For this review, take the finished solid that the model builds, in its own axes (mm). Face numbers are marked on the shaded views. A direction names the side the tool comes from. Give positions to 0.01 mm unless a question says otherwise; leave off trailing zeros. Write each loop counter-clockwise with the first axis right and the second up, starting at its lowest first coordinate (ties: lowest second). Pieces come first, ordered by that corner, then holes. Notation, with made-up numbers: M -31.75,33.5 L -14.75,33.5 A30 ccw -14.75,58.5 Z; hole C 28,58 d4. An arc over 180 degrees is marked long. One line per item, written item: value. Start each with the question number.
Item 1: Consider section A-A, the plane z = -4.1. Write out the cut boundary in (x, y), and give its area (3 significant figures).
Item 2: Mouldability with a two-part tool opening along X and no side actions: class the marked faces 4, 5, 6 and 7 as released by +X, released by -X, zero draft, split by the parting line, or undercut.
Item 3: To check wall thickness, follow probe 1 along X at (y, z) = (0.05, -5); probe 2 along Z at (x, y) = (0, 3.45); probe 3 along Y at (x, z) = (0.75, -7.5). State the ranges of each line that lie inside material, in increasing order.
Item 4: Consider section B-B, the plane y = 1.45. Write out the cut boundary in (x, z), and give its area (3 significant figures).
Item 5: Consider section C-C, the plane x = 2.5. Write out the cut boundary in (y, z), and give its area (3 significant figures).
Item 6: Clearance check with flat-ended pins moving along their axes: pin 1 Ø2 at (y, z) = (0.5, -2) entering from +X; pin 2 Ø1 at (y, z) = (2.5, -2) entering from -X; pin 3 Ø2 at (x, z) = (-2, -3.5) entering from +Y; pin 4 Ø1 at (x, z) = (6, -7) entering from +Y. State where each tip first meets the part, or that it passes through.
Item 7: Consider section D-D, the plane y = 2.7. Write out the cut boundary in (x, z).
Item 8: Tool access review of the marked faces 1, 2 and 3: name each direction out of +Z, -Z, +X, -X, +Y, -Y from which nothing blocks a thin tool from reaching the whole face with its end or side.
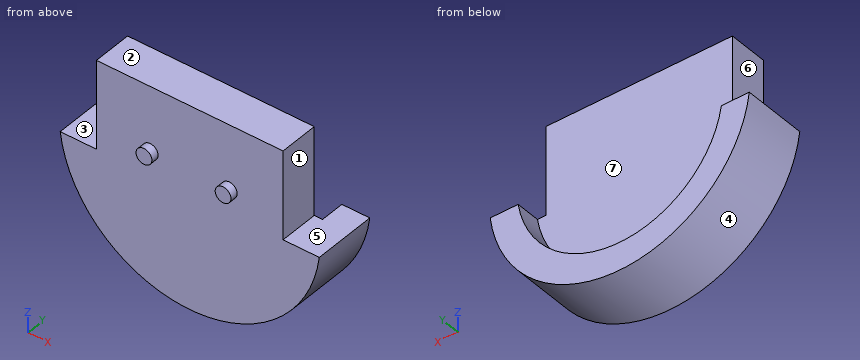
```python
from build123d import *

# Parameters (mm, degrees)
EXTRUDE_1_DEPTH = 2.5
EXTRUDE_2_DEPTH = 1.55
SKETCH_3_R      = 0.5
EXTRUDE_3_DEPTH = 0.5


with BuildPart() as part:
    # 草图1 → 凸台-拉伸1 (new body)
    with BuildSketch(Plane(origin=(0, 0, 0), x_dir=(1, 0, 0), z_dir=(0, 1, 0))):
        with BuildLine():
            Line((-5.9, 0), (5.9, 0))
            Line((5.9, 0), (5.9, 5.6))
            Line((5.9, 5.6), (8.189169677, 5.6))
            ThreePointArc((8.189169677, 5.6), (0, 12.85), (-8.189169677, 5.6))
            Line((-8.189169677, 5.6), (-5.9, 5.6))
            Line((-5.9, 5.6), (-5.9, 0))
        make_face()
    extrude(amount=EXTRUDE_1_DEPTH)

    # 草图2 → 凸台-拉伸2 (add)
    with BuildSketch(Plane(origin=(0, 2.5, 0), x_dir=(1, 0, 0), z_dir=(0, 1, 0))):
        with BuildLine():
            Line((-8.189169677, 5.6), (-6.422616289, 5.6))
            ThreePointArc((-6.422616289, 5.6), (0, 11.1), (6.422616289, 5.6))
            Line((6.422616289, 5.6), (8.189169677, 5.6))
            ThreePointArc((8.189169677, 5.6), (0, 12.85), (-8.189169677, 5.6))
        make_face()
    extrude(amount=EXTRUDE_2_DEPTH)

    # 草图3 → 凸台-拉伸3 (add)
    with BuildSketch(Plane.XZ):
        with Locations(Location((-2.5, -4.1, 0), (0, 0, 90))):
            Circle(SKETCH_3_R)
        with Locations(Location((2.5, -4.1, 0), (0, 0, 90))):
            Circle(SKETCH_3_R)
    extrude(amount=EXTRUDE_3_DEPTH)


solid = part.part
```
Model answer:
1. outline: M -5.9,0 L -3,0 L -3,-0.5 L -2,-0.5 L -2,0 L 2,0 L 2,-0.5 L 3,-0.5 L 3,0 L 5.9,0 L 5.9,2.5 L -5.9,2.5 Z
1. area: 30.5 mm2
2. face 4: split by the parting line
2. face 5: zero draft
2. face 6: released by -X
2. face 7: undercut
3. probe 1: x = -5.9 to 5.9
3. probe 2: z = -12.85 to -11.1
3. probe 3: y = 0 to 2.5
4. outline: M -8.19,-5.6 A8.25 ccw 8.19,-5.6 L 5.9,-5.6 L 5.9,0 L -5.9,0 L -5.9,-5.6 Z
4. area: 157 mm2
5. outline: M -0.5,-4.6 L 0,-4.6 L 0,-12.46 L 4.05,-12.46 L 4.05,-10.6 L 2.5,-10.6 L 2.5,0 L 0,0 L 0,-3.6 L -0.5,-3.6 Z
5. area: 34.5 mm2
6. pin 1: stops at x = 5.9
6. pin 2: stops at x = -5.9
6. pin 3: stops at y = 2.5
6. pin 4: stops at y = 4.05
7. outline: M -8.19,-5.6 A8.25 ccw 8.19,-5.6 L 6.42,-5.6 A6.5 cw -6.42,-5.6 Z
8. face 1: +Z, +X, +Y, -Y
8. face 2: +Z, +X, -X, +Y, -Y
8. face 3: +Z, -X, +Y, -Y
